from build123d import *

# Parameters (mm, degrees)
SKETCH1_R           = 2.6
SKETCH1_W           = 25
SKETCH1_H           = 18
BOSS_EXTRUDE1_DEPTH = 3


with BuildPart() as part:
    # Sketch1 → Boss-Extrude1 (new body)
    with BuildSketch(Plane(origin=(0, 0, 0), x_dir=(1, 0, 0), z_dir=(0, 1, 0))):
        with BuildLine():
            Line((-10.5, 13.5), (10.5, 13.5))
            ThreePointArc((10.5, 13.5), (19.692388155, 9.692388155), (23.5, 0.5))
            Line((23.5, 0.5), (23.5, -0.5))
            ThreePointArc((23.5, -0.5), (19.692388155, -9.692388155), (10.5, -13.5))
            Line((10.5, -13.5), (-10.5, -13.5))
            ThreePointArc((-10.5, -13.5), (-19.692388155, -9.692388155), (-23.5, -0.5))
            Line((-23.5, -0.5), (-23.5, 0.5))
            ThreePointArc((-23.5, 0.5), (-19.692388155, 9.692388155), (-10.5, 13.5))
        make_face()
        with Locations(Location((18.05, 0, 0), (0, 0, 270))):
            Circle(SKETCH1_R, mode=Mode.SUBTRACT)
        with Locations(Location((-18.05, 0, 0), (0, 0, 90))):
            Circle(SKETCH1_R, mode=Mode.SUBTRACT)
        Rectangle(SKETCH1_W, SKETCH1_H, mode=Mode.SUBTRACT)
    extrude(amount=BOSS_EXTRUDE1_DEPTH)


solid = part.part
Read the model definition and answer for the solid it produces. Units are mm, in the model's axes. A direction names the side the tool comes from. Round coordinates to 2 decimals unless told otherwise and drop trailing zeros. Write each loop counter-clockwise with the first axis right and the second up, starting at its lowest first coordinate (ties: lowest second). Pieces come first, ordered by that corner, then holes. Notation, with made-up numbers: (78, 75.5) - (86, 75.5) arc R13 ccw to (86, 86.5) - close; hole circle Ø9 at (86, 78). An arc over 180 degrees is marked (long way). Use a Markdown table: item, result.
(1) The part is cut by section C-C (y = 2.5). Write down the section's boundary in (x, z).
Reported:
| item | result |
|---|---|
| outline | (-23.5, -0.5) arc R13 ccw to (-10.5, -13.5) - (10.5, -13.5) arc R13 ccw to (23.5, -0.5) - (23.5, 0.5) arc R13 ccw to (10.5, 13.5) - (-10.5, 13.5) arc R13 ccw to (-23.5, 0.5) - close; hole circle Ø5.2 at (-18.05, 0); hole (-12.5, -9) - (12.5, -9) - (12.5, 9) - (-12.5, 9) - close; hole circle Ø5.2 at (18.05, 0) |
(2) Straight lines are drawn through the part: line 1 along X through (y, z) = (0.8, 0); line 2 along Z through (x, y) = (-9, 2.55); line 3 along X through (y, z) = (2.85, 1.75). For each, find the intervals that lie inside material, in ascending order. Write a range as [from, to].
Reported:
| item | result |
|---|---|
| line 1 | [-23.5, -20.65], [-15.45, -12.5], [12.5, 15.45], [20.65, 23.5] |
| line 2 | [-13.5, -9], [9, 13.5] |
| line 3 | [-23.44, -19.97], [-16.13, -12.5], [12.5, 16.13], [19.97, 23.44] |
(3) Each of these flat-tipped pins is pushed along its axis until it touches: pin 1 Ø4 at (x, z) = (18.05, 0) entering from -Y; pin 2 Ø0.9 at (y, z) = (2, 2) entering from +X; pin 3 Ø1.5 at (x, z) = (13, 9.5) entering from -Y; pin 4 Ø1.5 at (y, z) = (2, -7.5) entering from -X. Where does it stop, or does it pass through?
Reported:
| item | result |
|---|---|
| pin 1 | through |
| pin 2 | x = 23.46 |
| pin 3 | y = 0 |
| pin 4 | x = -21.9 |
(4) The part is cut by section D-D (z = 8). Write down the section's boundary in (x, y), then the cut area to 3 significant figures.
Reported:
| item | result |
|---|---|
| outline | (-21.12, 0) - (-12.5, 0) - (-12.5, 3) - (-21.12, 3) - close; (12.5, 0) - (21.12, 0) - (21.12, 3) - (12.5, 3) - close |
| area | 51.7 mm2 |
(5) The mould has two halves that part along Z. Classify faces 1 (the flat face through (23.5, 1, 0)), 2 (the cylindrical face through (19.591, 1.479, -9.793)), 3 (the cylindrical face through (-15.51, 1.48, 0.56)): released by +Z, released by -Z, zero draft, split by the parting line, or undercut.
Reported:
| item | result |
|---|---|
| face 1 | zero draft |
| face 2 | released by -Z |
| face 3 | undercut |
(6) Which of the six approach directions +Z, -Z, +X, -X, +Y, -Y give full straight-line access (tool end or side, diameter ignored) to faces 4 (the flat face through (12.5, 1, 0)), 5 (the flat face through (0.3, 3, -9.2))?
Reported:
| item | result |
|---|---|
| face 4 | +Y, -Y |
| face 5 | +Z, -Z, +X, -X, +Y |
(7) The part is cut by section B-B (z = 0). Write down the section's boundary in (x, y), then the cut area to 3 significant figures.
Reported:
| item | result |
|---|---|
| outline | (-23.5, 0) - (-20.65, 0) - (-20.65, 3) - (-23.5, 3) - close; (-15.45, 0) - (-12.5, 0) - (-12.5, 3) - (-15.45, 3) - close; (12.5, 0) - (15.45, 0) - (15.45, 3) - (12.5, 3) - close; (20.65, 0) - (23.5, 0) - (23.5, 3) - (20.65, 3) - close |
| area | 34.8 mm2 |
(8) The part is cut by section A-A (x = 6). Write down the section's boundary in (y, z), then the cut area to 3 significant figures.
Reported:
| item | result |
|---|---|
| outline | (0, -13.5) - (3, -13.5) - (3, -9) - (0, -9) - close; (0, 9) - (3, 9) - (3, 13.5) - (0, 13.5) - close |
| area | 27.0 mm2 |
